For this review, take the finished solid that the model builds, in its own axes (mm). A direction names the side the tool comes from. Round coordinates to 2 decimals unless told otherwise and drop trailing zeros. Order: outer loops, then holes, each group sorted by start corner. A loop starts at its lowest first (then second) coordinate and runs counter-clockwise, first axis right, second up. Notation, with made-up numbers: (-19, 55.25) -> (20, 55.25) arc R8 cw to (20, 63.25) -> close; hole circle Ø6 at (56.25, -23). An arc over 180 degrees is marked (long way). Use a Markdown table: item, result. Add a question column.
1) Wall thickness on line 1 along Y through (x, z) = (0, 3); line 2 along X through (y, z) = (0, 3.1); line 3 along Y through (x, z) = (-5, 1.6): over which ranges is each line inside the solid? List them lowest first. Write a range as [from, to].
2) Machinability: for faces 4 (the face through (-12, -8, 5)), 5 (the face through (15, 1, 3)), 6 (the face through (18.1, 0, 0.5)), which of the approach directions +Z, -Z, +X, -X, +Y, -Y give a long, thin tool a straight path to every point of the face, cutting with its end or side? Answer none if there is none.
3) Consider section A-A (y = -17). State the section outline as (x, z) points, plus the area to 3 significant figures.
4) Consider section B-B (z = 3). State the section outline as (x, y) points, plus the area to 3 significant figures.
5) Draft analysis for pull direction X (two halves, no side actions). For faces 1 (the face through (1.5, -16.2, 1)), 2 (the face through (-13.974, 0.847, 3.602)), 3 (the face through (-15.97, 0.98, 2.52)), state which applies: pulls with the +X half, pulls with the -X half, needs draft (parallel to the pull), parting line crosses it, or undercut.
6) Clearance check with flat-ended pins moving along their axes: P1, Ø6, axis at x = 17.5, y = -15.5, coming from the +Z side; P2, Ø3, axis at y = 4, z = 3.5, coming from the -X side; P3, Ø3, axis at y = -16.5, z = 1, coming from the +X side. State where each tip first meets the part, or that it passes through.
```python
from build123d import *

# Parameters (mm, degrees)
F1_ANGLE    = 358
F2_C1_SIZE2 = 4
F2_C1_SIZE  = 2
F2_C2_SIZE2 = 4
F2_C2_SIZE  = 2
F3_SIZE     = 1
F4_R        = 3
F5_T2_ANGLE = 359.64


# Not quite as in the source:
# - a fillet or chamfer that OpenCascade refuses, or shapes differently, is made with other operations: its cross-section is extruded or revolved along the edge and cut away or added


with BuildPart() as f1:
    # F0 (on Front) → F1 (revolve)
    with BuildSketch(Plane.XZ):
        Polygon((14, 0), (22, 0), (22, 1), (16, 1), (16, 5), (14, 5), align=None)
    revolve(axis=Axis((0, 0, -0.0525576656), (0, 0, 1)), revolution_arc=F1_ANGLE)

    # F2: chamfer of 4 x 2 on 2 edges, made by hand

    # F2_c1
    f2_c1_edges = [f1.edges().sort_by_distance(p)[0] for p in [
        (15, 0, 5),
    ]]
    f2_c1_side = f1.faces().sort_by_distance((15, 0.04, 5))[0]
    chamfer(f2_c1_edges, length=F2_C1_SIZE, length2=F2_C1_SIZE2, reference=f2_c1_side)

    # F2_c2
    f2_c2_edges = [f1.edges().sort_by_distance(p)[0] for p in [
        (14.9908624053, -0.5234924505, 5),
    ]]
    f2_c2_side = f1.faces().sort_by_distance((14.9894664254, -0.5634680836, 5))[0]
    chamfer(f2_c2_edges, length=F2_C2_SIZE, length2=F2_C2_SIZE2, reference=f2_c2_side)

    # F3
    f3_edges = [f1.edges().sort_by_distance(p)[0] for p in [
        (-13.997868, 0.244334, 0),
    ]]
    chamfer(f3_edges, length=F3_SIZE)

    # F4
    f4_edges = [f1.edges().sort_by_distance(p)[0] for p in [
        (-13.997868, 0.244334, 1),
    ]]
    fillet(f4_edges, radius=F4_R)

    # F5: chamfer of 1 x 0.5 on 1 edges, made by hand

    # F5_s1 → F5_t2 (revolve, cut)
    with BuildSketch(Plane(origin=(0, 0, 0), x_dir=(0, 0, 1), z_dir=(-0.0143112113, -0.9998975894, 0))):
        Polygon((5, -15.5), (4, -16), (5, -16), align=None)
    revolve(axis=Axis((0, 0, 5), (0, 0, 1)), revolution_arc=F5_T2_ANGLE, mode=Mode.SUBTRACT)


solid = f1.part
```
Results list:
| question | item | result |
|---|---|---|
| 1 | line 1 | [-16, -14], [14, 16] |
| 1 | line 2 | [-16, -14] |
| 1 | line 3 | [-15.2, -13.15], [13.15, 15.2] |
| 2 | face 4 | +Z, +X, -X, +Y, -Y |
| 2 | face 5 | +Z, +X |
| 2 | face 6 | +Z, -Z, +X |
| 3 | outline | (-13.96, 0) -> (13.96, 0) -> (13.96, 1) -> (-13.96, 1) -> close |
| 3 | area | 27.9 mm2 |
| 4 | outline | (13.92, -1.49) arc R14 cw (long way) to (13.96, 1) -> (15.97, 1) arc R16 ccw (long way) to (15.92, -1.56) -> close |
| 4 | area | 183 mm2 |
| 5 | face 1 | needs draft |
| 5 | face 2 | undercut |
| 5 | face 3 | parting line crosses it |
| 6 | P1 | z = 1 |
| 6 | P2 | x = -15.8 |
| 6 | P3 | x = 16.09 |
